from build123d import *

# Parameters (mm, degrees)
F0_R      = 7.9375
F1_DEPTH  = 1.5875
F2_R      = 6.35
F3_DEPTH  = 7
F4_R      = 6.35
F5_DEPTH  = 7
F6_R      = 9.587497
F7_DEPTH  = 1.5875
F8_R      = 9.587497
F9_DEPTH  = 1.5875
F10_R     = 9.587497
F10_R_2   = 8
F11_DEPTH = 5
F12_R     = 9.587497
F12_R_2   = 8
F13_DEPTH = 5
F14_R     = 4.087495
F15_DEPTH = 18.7625


with BuildPart() as f1:
    # F0 (on Top) → F1 (new body)
    with BuildSketch(Plane.XY):
        Circle(F0_R)
    extrude(amount=F1_DEPTH)

    # F2 (on face) → F3 (join)
    with BuildSketch(Plane.XY.offset(1.5875)):
        Circle(F2_R)
    extrude(amount=F3_DEPTH)

    # F4 (on face) → F5 (join)
    with BuildSketch(Plane(origin=(0, 0, 0), x_dir=(1, 0, 0), z_dir=(0, 0, -1))):
        Circle(F4_R)
    extrude(amount=F5_DEPTH)

    # F6 (on face) → F7 (join)
    with BuildSketch(Plane.XY.offset(8.5875)):
        Circle(F6_R)
    extrude(amount=F7_DEPTH)

    # F8 (on face) → F9 (join)
    with BuildSketch(Plane(origin=(0, 0, -7), x_dir=(1, 0, 0), z_dir=(0, 0, -1))):
        Circle(F8_R)
    extrude(amount=F9_DEPTH)

    # F10 (on face) → F11 (join)
    with BuildSketch(Plane(origin=(0, 0, -8.5875), x_dir=(1, 0, 0), z_dir=(0, 0, -1))):
        Circle(F10_R)
        Circle(F10_R_2, mode=Mode.SUBTRACT)
    extrude(amount=F11_DEPTH)

    # F12 (on face) → F13 (join)
    with BuildSketch(Plane.XY.offset(10.175)):
        Circle(F12_R)
        Circle(F12_R_2, mode=Mode.SUBTRACT)
    extrude(amount=F13_DEPTH)

    # F14 (on face) → F15 (cut, through all)
    with BuildSketch(Plane(origin=(0, 0, -8.5875), x_dir=(1, 0, 0), z_dir=(0, 0, -1))):
        Circle(F14_R)
    extrude(amount=-F15_DEPTH, mode=Mode.SUBTRACT)


solid = f1.part
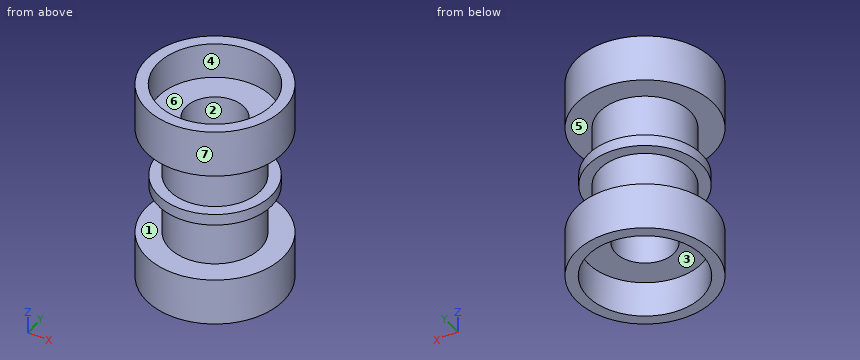
Input: part model. Units: mm. Frame: model coordinates. Face numbers are marked on the shaded views. A direction names the side the tool comes from. Round coordinates to 2 decimals unless told otherwise and drop trailing zeros. Loops run counter-clockwise (first coordinate to the right, second up) from the corner with the lowest first, then second, coordinate; pieces in that order, holes last. Notation, with made-up numbers: M 49,20 L 93,20 A20 cw 93,25 Z; hole C 81,35 d2. An arc over 180 degrees is marked long. Answer as CSV lines item,"result". Start each with the question number.
(1) Section D-D, the plane y = 7.25. Output: boundary loops of the cut face in (x, z) (1 decimal).
(2) Reachability of the marked faces 1, 2, 3 and 4 from +Z, -Z, +X, -X, +Y, -Y: full face, straight path, thin tool, end or side. Return the list, or none.
(3) Section C-C, the plane z = -1. Output: boundary loops of the cut face in (x, y), plus the area to 3 significant figures.
(4) First-contact query: pin 1 (5 mm diameter, centred on x = 2.5, y = 3, fed in from +Z) (3 decimals); pin 2 (2 mm diameter, centred on x = -6.5, z = -9.5, fed in from +Y); pin 3 (5 mm diameter, centred on x = 0, y = 3, fed in from -Z). Flat tips, straight axial feed; report the tip coordinate or a pass-through.
(5) Draft query along X for the marked faces 5, 6 and 7. Return one class per face: released by +X, released by -X, zero draft, split by the parting line, or undercut.
(6) Line query: line 1 (Z direction, x = -1.5, y = -7) (1 decimal); line 2 (Z direction, x = -2.25, y = -8.5) (1 decimal); line 3 (Y direction, x = 0, z = 6). Output: solid intervals per line, ascending. Write a range as [from, to].
Values found:
1,outline,"M -6.3,-13.6 L -3.4,-13.6 L -3.4,-8.6 L 3.4,-8.6 L 3.4,-13.6 L 6.3,-13.6 L 6.3,-7 L -6.3,-7 Z; M -6.3,8.6 L 6.3,8.6 L 6.3,15.2 L 3.4,15.2 L 3.4,10.2 L -3.4,10.2 L -3.4,15.2 L -6.3,15.2 Z; M -3.2,0 L 3.2,0 L 3.2,1.6 L -3.2,1.6 Z"
2,face 1,"none"
2,face 2,"+Z, -Z"
2,face 3,"-Z"
2,face 4,"+Z"
3,outline,"C 0,0 d12.7; hole C 0,0 d8.17"
3,area,"74.2 mm²"
4,pin 1,"stops at z = 10.175"
4,pin 2,"stops at y = 7.85"
4,pin 3,"stops at z = -8.59"
5,face 5,"zero draft"
5,face 6,"undercut"
5,face 7,"split by the parting line"
6,line 1,"z = [-8.6, -7], [0, 1.6], [8.6, 10.2]"
6,line 2,"z = [-13.6, -7], [8.6, 15.2]"
6,line 3,"y = [-6.35, -4.09], [4.09, 6.35]"
